Can you work these out from the drawing? Everything is in mm from the part's minimum corner. Round coordinates to 2 decimals unless told otherwise and drop trailing zeros. Order: outer loops, then holes, each group sorted by start corner. A loop starts at its lowest first (then second) coordinate and runs counter-clockwise, first axis right, second up. Notation, with made-up numbers: (-5, 27) -> (19, 27) arc R9 cw to (19, 37) -> close; hole circle Ø7 at (-29, 77.5). An arc over 180 degrees is marked (long way). Use a Markdown table: item, result. Add a question column.
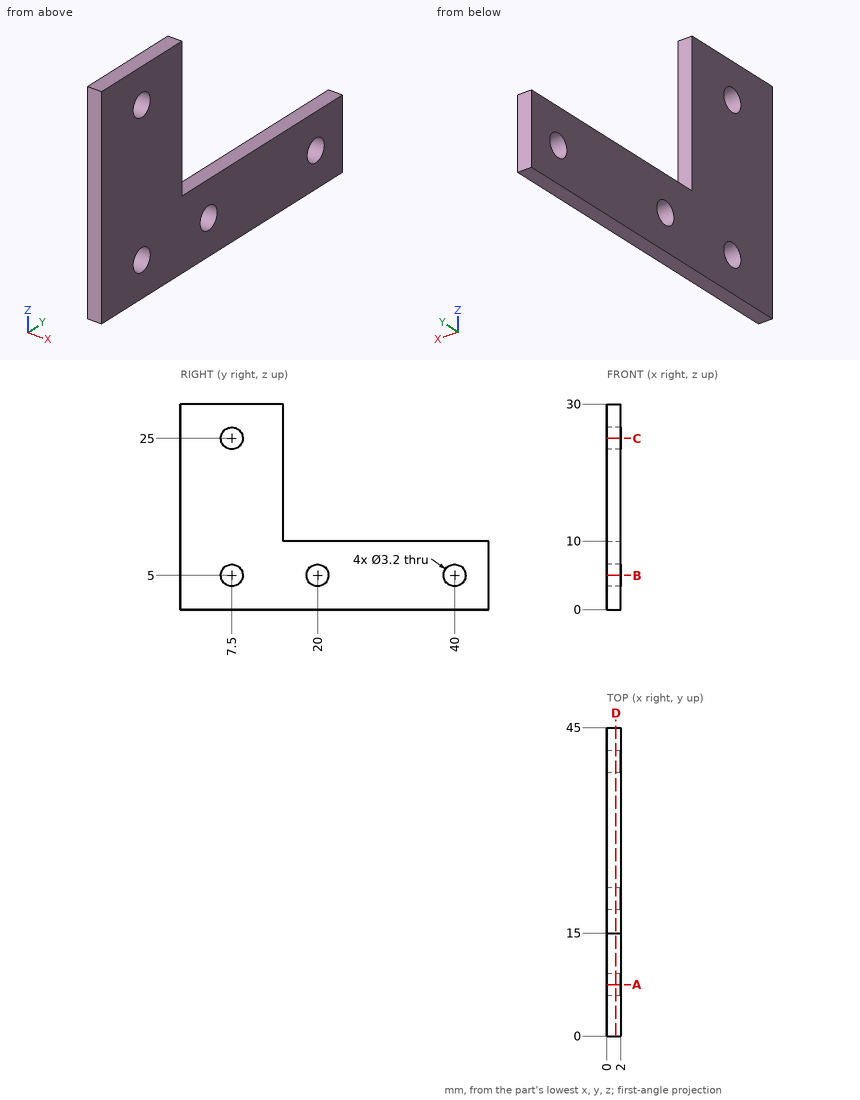
(1) I want a section at A-A on y = 7.5. List the corners of the cut face in (x, z) for me, and give its area (3 significant figures).
(2) Please list where these lines run through material, in increasing order: probe 1 along Z at (x, y) = (1.15, 7.5); probe 2 along Z at (x, y) = (0.55, 40); probe 3 along Z at (x, y) = (0.2, 7). Write a range as from..to.
(3) I want a section at D-D on x = 1.3. List the corners of the cut face in (y, z) for me.
(4) I'm going to push a flat-ended pin straight in: P1, Ø5, axis at y = 7.5, z = 5, coming from the +X side. Where does the tip first touch, or does it pass through?
(5) I want a section at C-C on z = 25. List the corners of the cut face in (x, y) for me.
(6) I want a section at B-B on z = 5. List the corners of the cut face in (x, y) for me, and give its area (3 significant figures).
Output:
| question | item | result |
|---|---|---|
| 1 | outline | (0, 0) -> (2, 0) -> (2, 3.4) -> (0, 3.4) -> close; (0, 6.6) -> (2, 6.6) -> (2, 23.4) -> (0, 23.4) -> close; (0, 26.6) -> (2, 26.6) -> (2, 30) -> (0, 30) -> close |
| 1 | area | 47.2 mm² |
| 2 | probe 1 | 0..3.4, 6.6..23.4, 26.6..30 |
| 2 | probe 2 | 0..3.4, 6.6..10 |
| 2 | probe 3 | 0..3.48, 6.52..23.48, 26.52..30 |
| 3 | outline | (0, 0) -> (45, 0) -> (45, 10) -> (15, 10) -> (15, 30) -> (0, 30) -> close; hole circle Ø3.2 at (7.5, 5); hole circle Ø3.2 at (7.5, 25); hole circle Ø3.2 at (20, 5); hole circle Ø3.2 at (40, 5) |
| 4 | P1 | x = 2 |
| 5 | outline | (0, 0) -> (2, 0) -> (2, 5.9) -> (0, 5.9) -> close; (0, 9.1) -> (2, 9.1) -> (2, 15) -> (0, 15) -> close |
| 6 | outline | (0, 0) -> (2, 0) -> (2, 5.9) -> (0, 5.9) -> close; (0, 9.1) -> (2, 9.1) -> (2, 18.4) -> (0, 18.4) -> close; (0, 21.6) -> (2, 21.6) -> (2, 38.4) -> (0, 38.4) -> close; (0, 41.6) -> (2, 41.6) -> (2, 45) -> (0, 45) -> close |
| 6 | area | 70.8 mm² |
